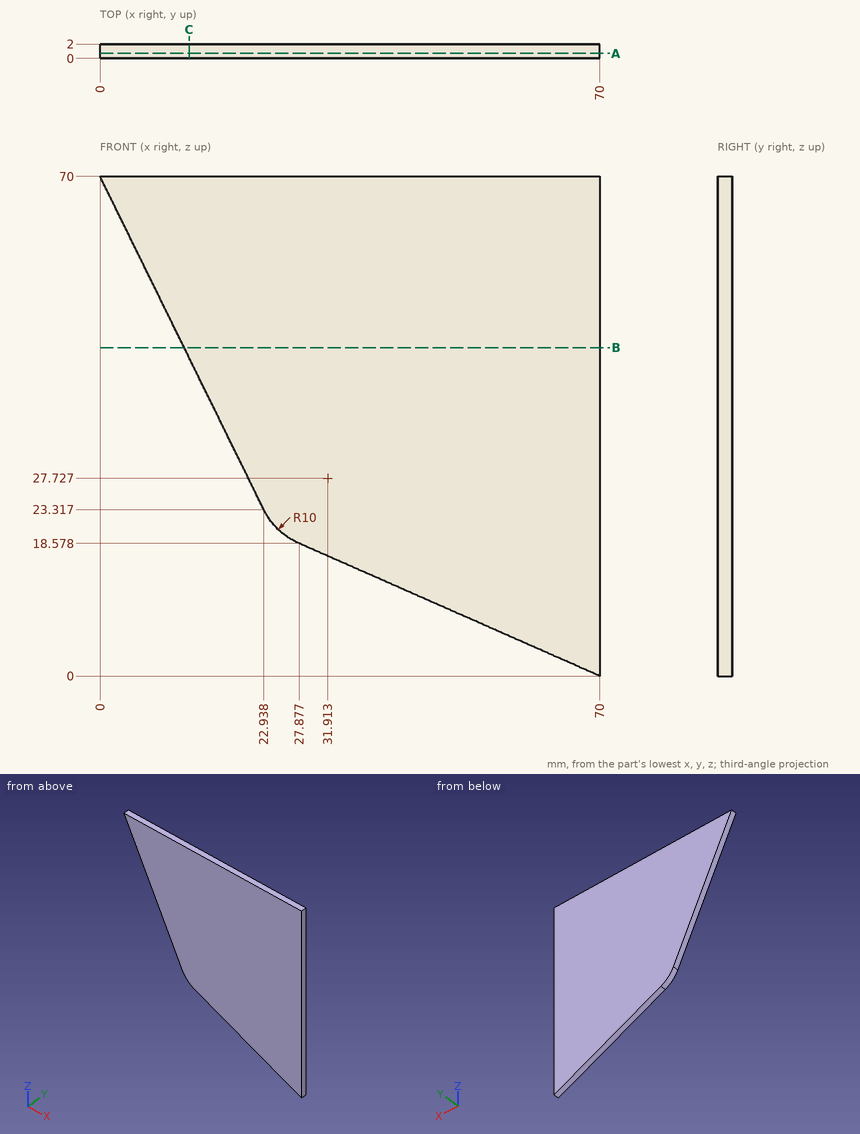
Geometry check sheet. Reference: drawing and pictorial views, mm from the part's lowest x, y, z. Round coordinates to 2 decimals unless told otherwise and drop trailing zeros. Write each loop counter-clockwise with the first axis right and the second up, starting at its lowest first coordinate (ties: lowest second). Pieces come first, ordered by that corner, then holes. Notation, with made-up numbers: (37, 71) -> (79, 71) arc R30 cw to (79, 93) -> close; hole circle Ø9 at (65, 41). An arc over 180 degrees is marked (long way). Answer as CSV lines item,"result". Start each with the question number.
1) Material ranges on line 1 (Z direction, x = 62.5, y = 1.35); line 2 (Z direction, x = 5.5, y = 0.5) (1 decimal); line 3 (X direction, y = 1.4, z = 5) (1 decimal), recorded low to high. Write a range as from..to.
2) Section check B-B on z = 46. Enter the section's corners in (x, y).
3) Section check C-C on x = 12.5. Enter the section's corners in (y, z).
4) Section check A-A on y = 0.7. Enter the section's corners in (x, z).
Found:
1,line 1,"z = 3.31..70"
1,line 2,"z = 58.8..70"
1,line 3,"x = 58.7..70"
2,outline,"(11.79, 0) -> (70, 0) -> (70, 2) -> (11.79, 2) -> close"
3,outline,"(0, 44.56) -> (2, 44.56) -> (2, 70) -> (0, 70) -> close"
4,outline,"(0, 70) -> (22.94, 23.32) arc R10 ccw to (27.88, 18.58) -> (70, 0) -> (70, 70) -> close"
